from build123d import *

# Parameters (mm, degrees)
SKETCH1_W           = 17.5
SKETCH1_H           = 5.2
SKETCH1_W_2         = 15.5
SKETCH1_H_2         = 3.2
BOSS_EXTRUDE1_DEPTH = 7.5
SKETCH2_W           = 17.5
SKETCH2_H           = 5.2
BOSS_EXTRUDE2_DEPTH = 1.5


with BuildPart() as part:
    # Sketch1 → Boss-Extrude1 (new body)
    with BuildSketch(Plane(origin=(0, 0, 0), x_dir=(1, 0, 0), z_dir=(0, 1, 0))):
        with Locations((7.75, 1.6)):
            Rectangle(SKETCH1_W, SKETCH1_H)
        with Locations((7.75, 1.6)):
            Rectangle(SKETCH1_W_2, SKETCH1_H_2, mode=Mode.SUBTRACT)
    extrude(amount=BOSS_EXTRUDE1_DEPTH)

    # Sketch2 → Boss-Extrude2 (add)
    with BuildSketch(Plane.XZ):
        with Locations((7.75, -1.6)):
            Rectangle(SKETCH2_W, SKETCH2_H)
    extrude(amount=BOSS_EXTRUDE2_DEPTH)


solid = part.part
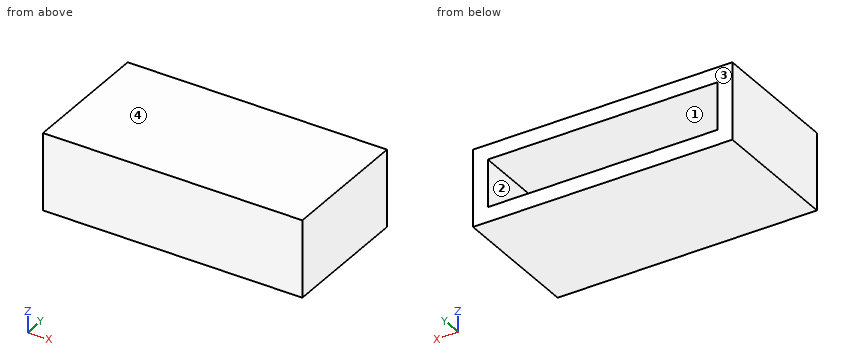
Can you work these out from the model? Positions are in its coordinate system, mm. Face numbers are marked on the shaded views. Coordinates: 2 decimals unless noted, no trailing zeros. Write each loop counter-clockwise with the first axis right and the second up, starting at its lowest first coordinate (ties: lowest second). Pieces come first, ordered by that corner, then holes. Notation, with made-up numbers: (48.5, 40) -> (59.5, 40) arc R22 cw to (59.5, 76) -> close; hole circle Ø9 at (-11.75, -19.75). An arc over 180 degrees is marked (long way). Write each question's results on one line, items separated by ' | '. Start each with the question number.
Item 1: I'm going to push a flat-ended pin straight in: P1, Ø2.5, axis at x = 11.5, z = -1.5, coming from the +Y side. Where does the tip first touch, or does it pass through?
Item 2: Please list where these lines run through material, in increasing order: probe 1 along Z at (x, y) = (0.25, 3.5); probe 2 along X at (y, z) = (7, -1.85); probe 3 along Y at (x, z) = (5.75, -1.9).
Item 3: Thinking about a two-plate mould opening in Z: for the marked faces 1, 2, 3 and 4, which applies, released by +Z, released by -Z, zero draft, split by the parting line, or undercut?
Item 4: If we section it at B-B, the plane z = -0.3: Write out the boundary of the cut face in (x, y), and give its area (4 significant figures).
Item 5: If we section it at A-A, the plane y = 5: Write out the boundary of the cut face in (x, z).
Item 6: If we section it at C-C, the plane x = 9.25: Write out the boundary of the cut face in (y, z), and give its area (3 significant figures).
Answer block:
1) P1: y = 0
2) probe 1: -4.2 to -3.2, 0 to 1 | probe 2: -1 to 0, 15.5 to 16.5 | probe 3: -1.5 to 0
3) face 1: undercut | face 2: undercut | face 3: zero draft | face 4: released by +Z
4) outline: (-1, -1.5) -> (16.5, -1.5) -> (16.5, 7.5) -> (15.5, 7.5) -> (15.5, 0) -> (0, 0) -> (0, 7.5) -> (-1, 7.5) -> close | area: 41.25 mm²
5) outline: (-1, -4.2) -> (16.5, -4.2) -> (16.5, 1) -> (-1, 1) -> close; hole (0, -3.2) -> (15.5, -3.2) -> (15.5, 0) -> (0, 0) -> close
6) outline: (-1.5, -4.2) -> (7.5, -4.2) -> (7.5, -3.2) -> (0, -3.2) -> (0, 0) -> (7.5, 0) -> (7.5, 1) -> (-1.5, 1) -> close | area: 22.8 mm²
